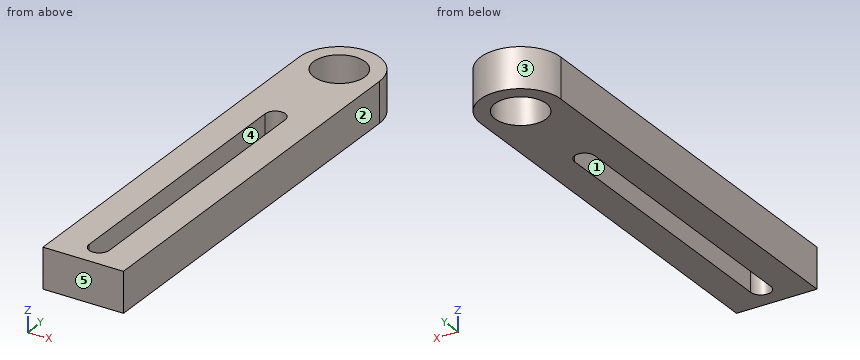
from build123d import *

# Parameters (mm, degrees)
F1_DEPTH = 8


with BuildPart() as f1:
    # F0 (on Top) → F1 (new body)
    with BuildSketch(Plane.XY):
        with BuildLine():
            ThreePointArc((-5.1, 0), (0, 5.1), (5.1, 0))
            Line((5.1, 0), (8, 0))
            ThreePointArc((8, 0), (0, 8), (-8, 0))
            Line((-8, 0), (-5.1, 0))
        make_face()
        with BuildLine():
            Line((8, 0), (5.1, 0))
            ThreePointArc((5.1, 0), (0, -5.1), (-5.1, 0))
            Line((-5.1, 0), (-8, 0))
            ThreePointArc((-8, 0), (0, -8), (8, 0))
        make_face()
        with BuildLine():
            Line((8, -80), (8, 0))
            ThreePointArc((8, 0), (0, -8), (-8, 0))
            Line((-8, 0), (-8, -80))
            Line((-8, -80), (8, -80))
        make_face()
        with BuildLine():
            ThreePointArc((-2, -20), (0, -18), (2, -20))
            Line((2, -20), (2, -75))
            ThreePointArc((2, -75), (0, -77), (-2, -75))
            Line((-2, -75), (-2, -20))
        make_face(mode=Mode.SUBTRACT)
    extrude(amount=F1_DEPTH)


solid = f1.part
Build history of the part. All positions in model axes, mm. Face numbers are marked on the shaded views. A direction names the side the tool comes from. Round coordinates to 2 decimals unless told otherwise and drop trailing zeros. Write each loop counter-clockwise with the first axis right and the second up, starting at its lowest first coordinate (ties: lowest second). Pieces come first, ordered by that corner, then holes. Notation, with made-up numbers: (30, 14) -> (75, 14) arc R25 cw to (75, 45) -> close; hole circle Ø9 at (8.25, 77.25). An arc over 180 degrees is marked (long way). Write item = value, one per line.
(1) Band-saw the part on B-B (x = 0). Give the cut face in (y, z).
Answer:
outline = (-80, 0) -> (-77, 0) -> (-77, 8) -> (-80, 8) -> close; (-18, 0) -> (-5.1, 0) -> (-5.1, 8) -> (-18, 8) -> close; (5.1, 0) -> (8, 0) -> (8, 8) -> (5.1, 8) -> close
(2) Band-saw the part on D-D (y = -1.5). Give the cut face in (x, z).
Answer:
outline = (-8, 0) -> (-4.87, 0) -> (-4.87, 8) -> (-8, 8) -> close; (4.87, 0) -> (8, 0) -> (8, 8) -> (4.87, 8) -> close
(3) Flat gauge pins, fed straight in: pin 1 (4 mm diameter, centred on x = 4.5, z = 2, fed in from +Y); pin 2 (8 mm diameter, centred on x = 0, y = 0, fed in from -Z). Where does each tip first touch, or does it go through?
Answer:
pin_1 = 7.6
pin_2 = through
(4) Band-saw the part on A-A (y = -36). Give the cut face in (x, z).
Answer:
outline = (-8, 0) -> (-2, 0) -> (-2, 8) -> (-8, 8) -> close; (2, 0) -> (8, 0) -> (8, 8) -> (2, 8) -> close
(5) Probe L1, parallel to Y at x = 0, z = 4.5; L2, parallel to X at y = -38, z = 4.75; L3, parallel to Y at x = 1.25, z = 3.25. List the from-to ranges inside material, lowest first.
Answer:
L1 = -80 to -77, -18 to -5.1, 5.1 to 8
L2 = -8 to -2, 2 to 8
L3 = -80 to -76.56, -18.44 to -4.94, 4.94 to 7.9
(6) Tool access for the marked faces 1 and 2: list every direction of +Z, -Z, +X, -X, +Y, -Y with a clear straight run to the whole face (end or side of a thin tool).
Answer:
face_1 = +Z, -Z
face_2 = +Z, -Z, +X, +Y, -Y
(7) Band-saw the part on C-C (z = 3). Give the cut face in (x, y), then the cut area to 3 significant figures.
Answer:
outline = (-8, -80) -> (8, -80) -> (8, 0) arc R8 ccw to (-8, 0) -> close; hole circle Ø10.2 at (0, 0); hole (-2, -75) arc R2 ccw to (2, -75) -> (2, -20) arc R2 ccw to (-2, -20) -> close
area = 1,070 mm2
(8) Two-plate mould, pull along X, no slides. Class the marked faces 3, 4 and 5: pulls with the +X half, pulls with the -X half, needs draft (parallel to the pull), parting line crosses it, or undercut.
Answer:
face_3 = parting line crosses it
face_4 = undercut
face_5 = needs draft
